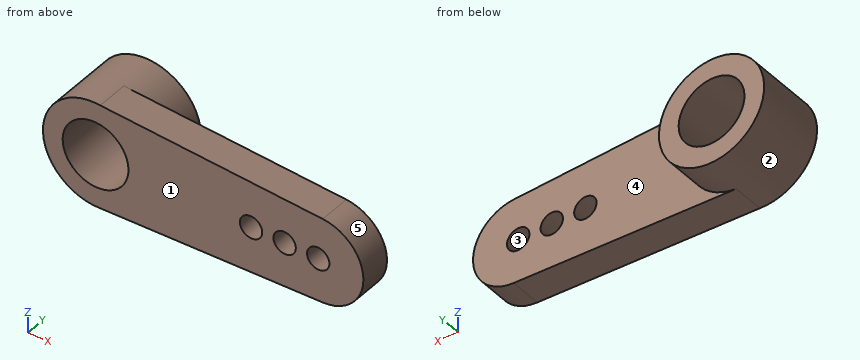
from build123d import *

# Parameters (mm, degrees)
SKETCH1_R           = 2.9845
SKETCH1_R_2         = 1.8669
BOSS_EXTRUDE1_DEPTH = 3.9878
BOSS_EXTRUDE2_DEPTH = 1.778
SKETCH3_R           = 0.635
CUT_EXTRUDE1_DEPTH  = 16.994250438


with BuildPart() as part:
    # Sketch1 → Boss-Extrude1 (new body)
    with BuildSketch(Plane(origin=(0, 0, 0), x_dir=(1, 0, 0), z_dir=(0, 1, 0))):
        with Locations(Location((0, 0, 0), (0, 0, 270))):
            Circle(SKETCH1_R)
        with Locations(Location((0, 0, 0), (0, 0, 270))):
            Circle(SKETCH1_R_2, mode=Mode.SUBTRACT)
    extrude(amount=BOSS_EXTRUDE1_DEPTH)

    # Sketch2 → Boss-Extrude2 (add)
    with BuildSketch(Plane.XZ):
        with BuildLine():
            Line((12.8905, 2.413), (0.264116324, 2.972790409))
            ThreePointArc((0.264116324, 2.972790409), (2.201760139, 2.01481824), (2.9845, 0))
            ThreePointArc((2.9845, 0), (2.201760139, -2.01481824), (0.264116324, -2.972790409))
            Line((0.264116324, -2.972790409), (12.8905, -2.413))
            ThreePointArc((12.8905, -2.413), (15.198890025, 0), (12.8905, 2.413))
        make_face()
    extrude(amount=-BOSS_EXTRUDE2_DEPTH)

    # Sketch3 → Cut-Extrude1 (cut, through all)
    with BuildSketch(Plane.XZ):
        with Locations(Location((8.823490025, 0, 0), (0, 0, 270))):
            Circle(SKETCH3_R)
        with Locations(Location((10.728490025, 0, 0), (0, 0, 270))):
            Circle(SKETCH3_R)
        with Locations(Location((12.633490025, 0, 0), (0, 0, 270))):
            Circle(SKETCH3_R)
    extrude(amount=-CUT_EXTRUDE1_DEPTH, mode=Mode.SUBTRACT)


solid = part.part
Read the model definition and answer for the solid it produces. Units are mm, in the model's axes. Face numbers are marked on the shaded views. A direction names the side the tool comes from. Give positions to 0.01 mm unless a question says otherwise; leave off trailing zeros. Loops run counter-clockwise (first coordinate to the right, second up) from the corner with the lowest first, then second, coordinate; pieces in that order, holes last. Notation, with made-up numbers: (88, 73) - (127, 73) arc R36 ccw to (127, 111) - close; hole circle Ø4 at (20.5, 82.5). An arc over 180 degrees is marked (long way). Answer as CSV lines item,"result". Start each with the question number.
1) Determine the mould class of the marked faces 3, 4 and 5 for opening direction X: released by +X, released by -X, zero draft, split by the parting line, or undercut.
2) Straight lines are drawn through the part: L1, parallel to X at y = 1.25, z = 0; L2, parallel to X at y = 1.15, z = 0.55; L3, parallel to Y at x = 4.5, z = 1.3. For each, find the intervals that lie inside material, in ascending order. Write a range as from..to.
3) Each of these flat-tipped pins is pushed along its axis until it touches: pin 1 Ø1.7 at (x, z) = (12.63, 0) entering from +Y; pin 2 Ø1.5 at (x, y) = (1.5, 3) entering from +Z; pin 3 Ø1 at (x, y) = (8.5, 2) entering from -Z. Where does it stop, or does it pass through?
4) Find section A-A (z = 0). Write down the section's boundary in (x, y), then the cut area to 3 significant figures.
5) Find section B-B (x = 0). Write down the section's boundary in (y, z), then the cut area to 3 significant figures.
6) Which of the six approach directions +Z, -Z, +X, -X, +Y, -Y give full straight-line access (tool end or side, diameter ignored) to the marked faces 1 and 2?
7) Find section D-D (y = 3.15). Write down the section's boundary in (x, z), then the cut area to 3 significant figures.
8) Find section C-C (z = 0.85). Write down the section's boundary in (x, y), then the cut area to 3 significant figures.
Findings below:
1,face 3,"undercut"
1,face 4,"zero draft"
1,face 5,"released by +X"
2,L1,"-2.98..-1.87, 1.87..8.19, 9.46..10.09, 11.36..12, 13.27..15.2"
2,L2,"-2.93..-1.78, 1.78..8.51, 9.14..10.41, 11.05..12.32, 12.95..15.14"
2,L3,"0..1.78"
3,pin 1,"y = 1.78"
3,pin 2,"z = 2.89"
3,pin 3,"z = -2.63"
4,outline,"(-2.98, 0) - (-1.87, 0) - (-1.87, 3.99) - (-2.98, 3.99) - close; (1.87, 0) - (8.19, 0) - (8.19, 1.78) - (2.98, 1.78) - (2.98, 3.99) - (1.87, 3.99) - close; (9.46, 0) - (10.09, 0) - (10.09, 1.78) - (9.46, 1.78) - close; (11.36, 0) - (12, 0) - (12, 1.78) - (11.36, 1.78) - close; (13.27, 0) - (15.2, 0) - (15.2, 1.78) - (13.27, 1.78) - close"
4,area,"23.9 mm^2"
5,outline,"(0, -2.98) - (3.99, -2.98) - (3.99, -1.87) - (0, -1.87) - close; (0, 1.87) - (3.99, 1.87) - (3.99, 2.98) - (0, 2.98) - close"
5,area,"8.91 mm^2"
6,face 1,"+Z, -Z, +X, -X, -Y"
6,face 2,"+Y"
7,outline,"circle Ø5.97 at (0, 0); hole circle Ø3.73 at (0, 0)"
7,area,"17.0 mm^2"
8,outline,"(-2.86, 0) - (-1.66, 0) - (-1.66, 3.99) - (-2.86, 3.99) - close; (1.66, 0) - (15.04, 0) - (15.04, 1.78) - (2.86, 1.78) - (2.86, 3.99) - (1.66, 3.99) - close"
8,area,"31.2 mm^2"
